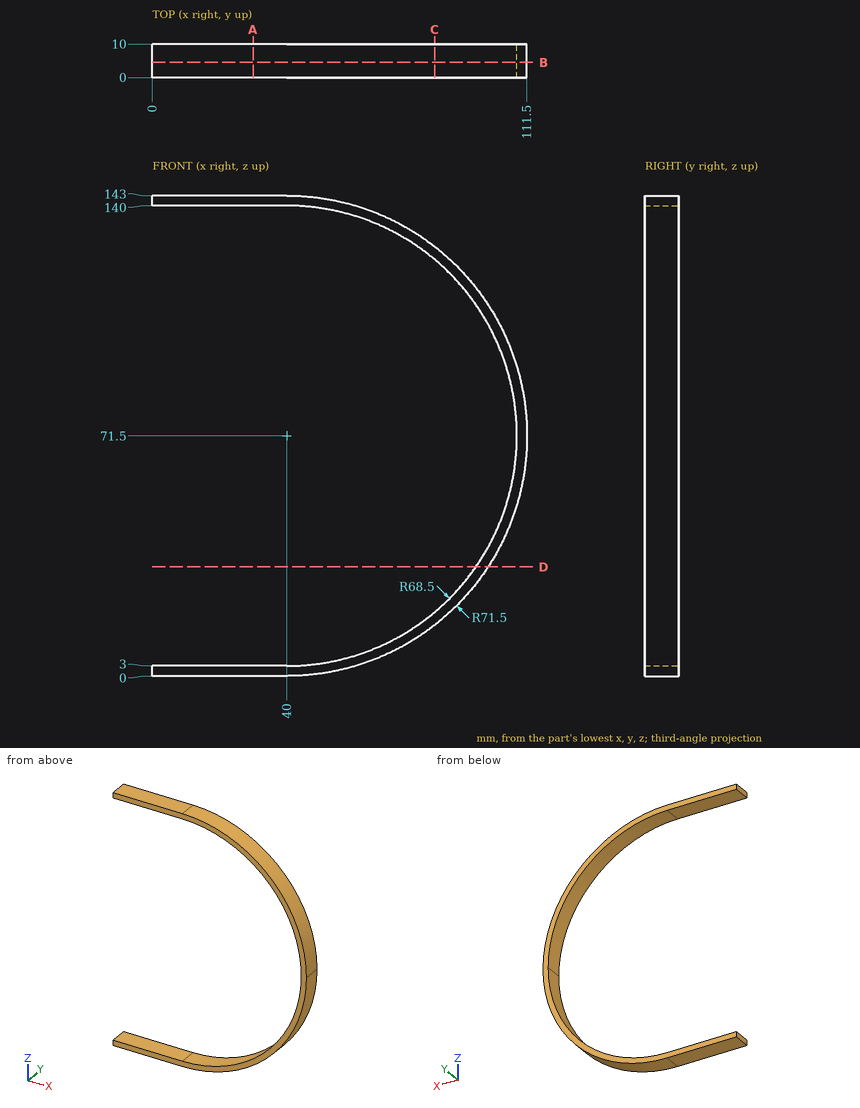
The figure shows three views and two pictorial views of one solid part (mm, origin at its lowest corner). Answer the questions. Give positions to 0.01 mm unless a question says otherwise; leave off trailing zeros. Order: outer loops, then holes, each group sorted by start corner. A loop starts at its lowest first (then second) coordinate and runs counter-clockwise, first axis right, second up. Notation, with made-up numbers: (-11, -3) -> (47, -3) arc R27 ccw to (47, 29) -> close; hole circle Ø6 at (26.5, -28.75). An arc over 180 degrees is marked (long way). Answer as CSV lines item,"result". Start each with the question number.
(1) Section D-D, the plane z = 32.5 is taken. Write down the section's boundary in (x, y), plus the area to 3 significant figures.
(2) Section B-B, the plane y = 4.5 is taken. Write down the section's boundary in (x, z), plus the area to 3 significant figures.
(3) Section C-C, the plane x = 84 is taken. Write down the section's boundary in (y, z).
(4) Consider line 1 along Z through (x, y) = (29.5, 3); line 2 along Z through (x, y) = (99.5, 5); line 3 along X through (y, z) = (1.75, 73). Determine where each line is inside the solid, lowest interval first.
(5) Each of these flat-tipped pins is pushed along its axis until it touches: pin 1 Ø1.5 at (y, z) = (3, 32.5) entering from +X; pin 2 Ø5 at (x, y) = (85.5, 1.5) entering from +Z; pin 3 Ø2 at (x, y) = (78, 4) entering from -Z. Where does it stop, or does it pass through?
(6) Section A-A, the plane x = 30 is taken. Write down the section's boundary in (y, z).
Entries:
1,outline,"(96.31, 0) -> (99.93, 0) -> (99.93, 10) -> (96.31, 10) -> close"
1,area,"36.1 mm²"
2,outline,"(0, 0) -> (40, 0) arc R71.5 ccw to (40, 143) -> (0, 143) -> (0, 140) -> (40, 140) arc R68.5 cw to (40, 3) -> (0, 3) -> close"
2,area,"900 mm²"
3,outline,"(0, 15.14) -> (10, 15.14) -> (10, 19) -> (0, 19) -> close; (0, 124) -> (10, 124) -> (10, 127.86) -> (0, 127.86) -> close"
4,line 1,"0 to 3, 140 to 143"
4,line 2,"31.85 to 37.56, 105.44 to 111.15"
4,line 3,"108.48 to 111.48"
5,pin 1,"x = 100.41"
5,pin 2,"z = 128.62"
5,pin 3,"z = 10.32"
6,outline,"(0, 0) -> (10, 0) -> (10, 3) -> (0, 3) -> close; (0, 140) -> (10, 140) -> (10, 143) -> (0, 143) -> close"
